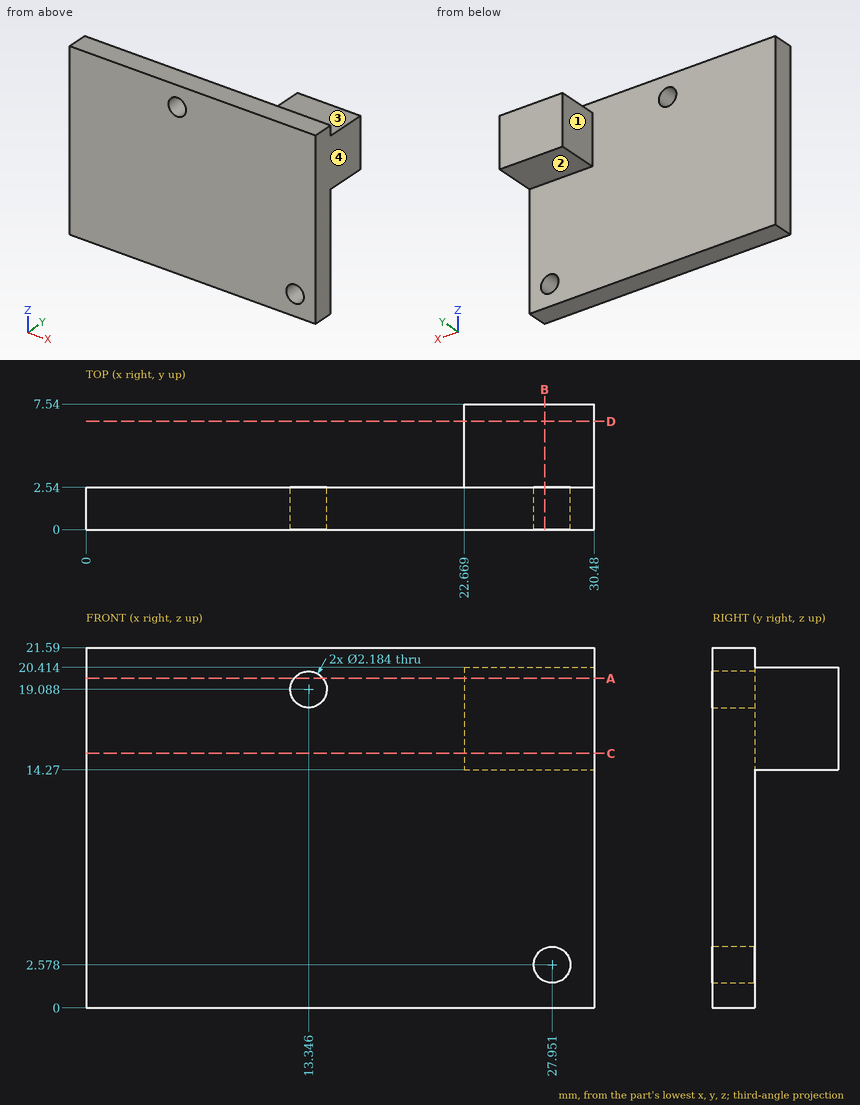
Check sheet for the drawn part. Datum: minimum x, y, z corner. Units: mm. A direction names the side the tool comes from. Round coordinates to 2 decimals unless told otherwise and drop trailing zeros. Order: outer loops, then holes, each group sorted by start corner. A loop starts at its lowest first (then second) coordinate and runs counter-clockwise, first axis right, second up.
(1) Access from +Z, -Z, +X, -X, +Y, -Y to the whole of each face (thin tool, end or side, straight path). Record for the marked faces 1, 2, 3 and 4.
(2) Cross-section at A-A, the plane z = 19.75. Enter the section's corners in (x, y) (1 decimal).
(3) Cross-section at B-B, the plane x = 27.5. Enter the section's corners in (y, z) (1 decimal).
(4) Go/stop test with flat-tipped pins: P1, Ø1.5, axis at x = 21.5, z = 13, coming from the +Y side; P2, Ø4, axis at y = 4.5, z = 16, coming from the -X side; P3, Ø1.5, axis at x = 28.5, y = 4, coming from the -Z side. Record where each tip stops, or that it passes through.
(5) Cross-section at D-D, the plane y = 6.5. Enter the section's corners in (x, z) (1 decimal), and give its area (3 significant figures).
(6) Scan lines: probe 1 along Z at (x, y) = (25.5, 6) (1 decimal); probe 2 along X at (y, z) = (5.25, 17.5); probe 3 along Y at (x, z) = (2, 9.75). Record each from-to range of solid material in increasing order.
(7) Cross-section at C-C, the plane z = 15.25. Enter the section's corners in (x, y).
Check sheet entries:
1. face 1: +Z, -Z, -X, +Y
1. face 2: -Z, +X, -X, +Y
1. face 3: +Z, +X, -X, +Y
1. face 4: +Z, -Z, +X, +Y, -Y
2. outline: (0, 0) - (12.5, 0) - (12.5, 2.5) - (0, 2.5) - close; (14.2, 0) - (30.5, 0) - (30.5, 7.5) - (22.7, 7.5) - (22.7, 2.5) - (14.2, 2.5) - close
3. outline: (0, 0) - (2.5, 0) - (2.5, 1.6) - (0, 1.6) - close; (0, 3.6) - (2.5, 3.6) - (2.5, 14.3) - (7.5, 14.3) - (7.5, 20.4) - (2.5, 20.4) - (2.5, 21.6) - (0, 21.6) - close
4. P1: stops at y = 2.54
4. P2: stops at x = 0
4. P3: stops at z = 14.27
5. outline: (22.7, 14.3) - (30.5, 14.3) - (30.5, 20.4) - (22.7, 20.4) - close
5. area: 48.0 mm2
6. probe 1: z = 14.3 to 20.4
6. probe 2: x = 22.67 to 30.48
6. probe 3: y = 0 to 2.54
7. outline: (0, 0) - (30.48, 0) - (30.48, 7.54) - (22.67, 7.54) - (22.67, 2.54) - (0, 2.54) - close
